Build history of the part. All positions in model axes, mm. Face numbers are marked on the shaded views. A direction names the side the tool comes from. Round coordinates to 2 decimals unless told otherwise and drop trailing zeros. Loops run counter-clockwise (first coordinate to the right, second up) from the corner with the lowest first, then second, coordinate; pieces in that order, holes last. Notation, with made-up numbers: (23.5, 37.5) - (43.5, 37.5) arc R25 ccw to (43.5, 72.5) - close; hole circle Ø4 at (56.25, -33). An arc over 180 degrees is marked (long way). Answer as CSV lines item,"result". Start each with the question number.
```python
from build123d import *

# Parameters (mm, degrees)
BASPROSKE_W     = 30
BASPROSKE_H     = 27.5
TOOTHCUT_DEPTH  = 50.117206761
TEETHCUTS_COUNT = 20
TEETHCUTS_ANGLE = 342
BORSKE_R        = 7.55
BORE_DEPTH      = 50.000508
SCALE1_SCALE    = 0.8


with BuildPart() as part:
    # BasProSke → Base-Revolve (revolve)
    with BuildSketch(Plane(origin=(0, 0, 0), x_dir=(1, 0, 0), z_dir=(0, 1, 0)), mode=Mode.PRIVATE) as base_revolve_sk:
        with Locations((15, 13.75)):
            Rectangle(BASPROSKE_W, BASPROSKE_H)
    revolve(base_revolve_sk.sketch.rotate(Axis((-10, 0, 0), (1, 0, 0)), 180), axis=Axis((-10, 0, 0), (1, 0, 0)))

    # TooCutSke → ToothCut (cut, through all)
    with BuildSketch(Plane(origin=(0, 0, 0), x_dir=(0, 0, -1), z_dir=(1, 0, 0))):
        with BuildLine():
            ThreePointArc((1.237725267, 21.838954008), (0, 21.874), (-1.237725267, 21.838954008))
            ThreePointArc((-1.237725267, 21.838954008), (-2.095118569, 24.870704072), (-3.853229952, 27.485216662))
            ThreePointArc((-3.853229952, 27.485216662), (0, 27.754), (3.853229952, 27.485216662))
            ThreePointArc((3.853229952, 27.485216662), (2.095118569, 24.870704072), (1.237725267, 21.838954008))
        make_face()
    toothcut = extrude(amount=TOOTHCUT_DEPTH, mode=Mode.SUBTRACT)

    # TeethCuts: ToothCut ×20 about axis
    teethcuts_axis = Axis((-10, 0, 0), (1, 0, 0))
    for i in range(1, TEETHCUTS_COUNT):
        add(toothcut.rotate(teethcuts_axis, i * TEETHCUTS_ANGLE / (TEETHCUTS_COUNT - 1)), mode=Mode.SUBTRACT)

    # BorSke → Bore (cut, symmetric)
    with BuildSketch(Plane(origin=(0, 0, 0), x_dir=(0, 0, -1), z_dir=(1, 0, 0))):
        with Locations(Location((0, 0, 0), (0, 0, 180))):
            Circle(BORSKE_R)
    extrude(amount=BORE_DEPTH, both=True, mode=Mode.SUBTRACT)


with BuildPart() as part_1:
    # Scale1: scaled about (15, 0, 0)
    add(part.part.scale(SCALE1_SCALE).moved(Location((3, 0, 0))))


solid = part_1.part
```
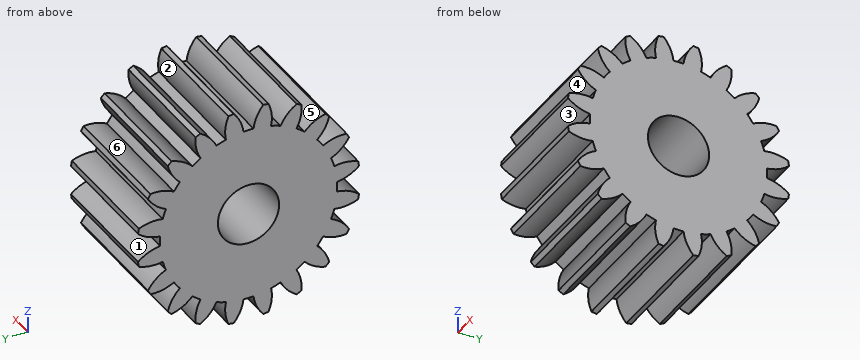
Q1. Band-saw the part on C-C, the plane z = 12. List the corners of the cut face in (x, y), then the cut area to 3 significant figures.
Q2. Band-saw the part on A-A, the plane z = 0. List the corners of the cut face in (x, y), then the cut area to 3 significant figures.
Q3. Pin check, flat tips, straight feed: pin 1 Ø4 at (x, z) = (12, -17) entering from +Y; pin 2 Ø4 at (x, y) = (21.5, -9.5) entering from -Z; pin 3 Ø2 at (x, y) = (23.5, 4) entering from +Z. Stop position of each tip, or through.
Q4. Tool access for the marked faces 4, 5 and 6: list every direction of +Z, -Z, +X, -X, +Y, -Y with a clear straight run to the whole face (end or side of a thin tool).
Q5. Wall check: probe 1 along Z at (x, y) = (18.5, -15); probe 2 along Z at (x, y) = (9, 18); probe 3 along Z at (x, y) = (24.5, -14). Give the ranges that are in metal, low to high. Write a range as [from, to].
Q6. Two-plate mould, pull along Y, no slides. Class the marked faces 1, 2 and 3: released by +Y, released by -Y, zero draft, split by the parting line, or undercut.
Q7. Band-saw the part on D-D, the plane y = -7. List the corners of the cut face in (x, z), then the cut area to 3 significant figures.
Reported:
1,outline,"(3, -14.41) - (27, -14.41) - (27, 14.41) - (3, 14.41) - close"
1,area,"692 mm2"
2,outline,"(3, -17.5) - (27, -17.5) - (27, -6.04) - (3, -6.04) - close; (3, 6.04) - (27, 6.04) - (27, 17.5) - (3, 17.5) - close"
2,area,"550 mm2"
3,pin 1,"stops at y = 15.93"
3,pin 2,"stops at z = -19.84"
3,pin 3,"stops at z = 21.79"
4,face 4,"+X, -X, -Y"
4,face 5,"+Z, +X, -X"
4,face 6,"+X, -X"
5,probe 1,"z = [-15.88, -12.86], [-9.62, 9.62], [12.86, 15.88]"
5,probe 2,"z = [-10.47, -7.39], [-4.6, -1.07], [1.07, 4.6], [7.39, 10.47]"
5,probe 3,"z = [-15.56, -11.52], [-10.5, 10.5], [11.52, 15.56]"
6,face 1,"released by +Y"
6,face 2,"undercut"
6,face 3,"released by -Y"
7,outline,"(3, -17.47) - (27, -17.47) - (27, 17.47) - (3, 17.47) - close"
7,area,"839 mm2"
